from build123d import *

# Parameters (mm, degrees)
SKETCH1_W                = 120
SKETCH1_H                = 30
BOSS_EXTRUDE1_DEPTH      = 100
CUT_EXTRUDE1_DEPTH       = 121.415945788
CUT_EXTRUDE1_DEPTH_BACK  = 121.415945788
SKETCH2_R                = 2.15
SKETCH2_W                = 20.1
SKETCH2_H                = 40.4
SKETCH3_OUTSIDE_W        = 153.812
SKETCH3_OUTSIDE_H        = 133.812
CUT_EXTRUDE2_DEPTH       = 121.415945788
CUT_EXTRUDE3_START       = -30
CUT_EXTRUDE3_DEPTH       = 30
SKETCH5_W                = 67.698745078
SKETCH5_H                = 100.8
CUT_EXTRUDE4_DEPTH       = 26
RIB1_REACH               = 122.416
SKETCH6_WALL_W           = 284.590065176
SKETCH6_WALL_H           = 4
RIB6_REACH               = 122.416
SKETCH7_WALL_W           = 284.590065176
SKETCH7_WALL_H           = 4
BOSS_EXTRUDE2_DEPTH      = 5
BOSS_EXTRUDE2_DEPTH_BACK = 4
SKETCH8_R                = 2.15
CUT_EXTRUDE5_DEPTH       = 84.326168543
CUT_EXTRUDE5_DEPTH_BACK  = 84.326168543
SKETCH9_R                = 2.75
SKETCH10_R               = 5
CUT_EXTRUDE6_DEPTH       = 3
CHAMFER1_SIZE            = 8
CUT_EXTRUDE7_START       = -12.194246874
CUT_EXTRUDE7_DEPTH       = 12.194246874
SKETCH12_W               = 37.282730079
SKETCH12_H               = 58.292887361
CUT_EXTRUDE8_DEPTH       = 108.591821251
SKETCH13_W               = 20.1
SKETCH13_H               = 40.4
BOSS_EXTRUDE3_DEPTH      = 4
SKETCH16_W               = 60
SKETCH16_H               = 40
BOSS_EXTRUDE4_DEPTH      = 4
CUT_EXTRUDE9_DEPTH       = 109.484577329
CUT_EXTRUDE9_DEPTH_BACK  = 109.484577329
SKETCH14_R               = 2.75
SKETCH15_R               = 5
CUT_EXTRUDE10_DEPTH      = 2
CHAMFER2_SIZE            = 0.2
CHAMFER3_SIZE            = 10
CUT_EXTRUDE11_DEPTH      = 109.484577329
CUT_EXTRUDE11_DEPTH_BACK = 109.484577329
CHAMFER4_SIZE            = 10


# Read off the part's stored shape, not the designer's step: Cut-Extrude3, Cut-Extrude7
with BuildPart() as part:
    # Sketch1 → Boss-Extrude1 (new body)
    with BuildSketch(Plane(origin=(0, 0, 0), x_dir=(1, 0, 0), z_dir=(0, 1, 0))):
        with Locations((0, -15)):
            Rectangle(SKETCH1_W, SKETCH1_H)
    extrude(amount=BOSS_EXTRUDE1_DEPTH)

    # Sketch2 → Cut-Extrude1 (cut, two sides: drawn at the far end of the back side and taken through both)
    with BuildSketch(Plane.XY.offset(30).offset(-CUT_EXTRUDE1_DEPTH_BACK)):
        with Locations((-4.95, 82.583541889)):
            Circle(SKETCH2_R)
        with Locations((4.95, 82.583541889)):
            Circle(SKETCH2_R)
        with Locations((-4.95, 34.383541889)):
            Circle(SKETCH2_R)
        with Locations((4.95, 34.383541889)):
            Circle(SKETCH2_R)
        with Locations((0, 58.483541889)):
            Rectangle(SKETCH2_W, SKETCH2_H)
    extrude(amount=CUT_EXTRUDE1_DEPTH + CUT_EXTRUDE1_DEPTH_BACK, mode=Mode.SUBTRACT)

    # Sketch3 outside → Cut-Extrude2 (cut, through all)
    with BuildSketch(Plane.XY.offset(30)):
        with Locations((0, 50)):
            Rectangle(SKETCH3_OUTSIDE_W, SKETCH3_OUTSIDE_H)
        with BuildLine():
            Line((-45, 23.283541889), (45, 23.283541889))
            Line((45, 23.283541889), (19.804596008, 86.568297014))
            ThreePointArc((19.804596008, 86.568297014), (0, 100), (-19.804596008, 86.568297014))
            Line((-19.804596008, 86.568297014), (-45, 23.283541889))
        make_face(mode=Mode.SUBTRACT)
    extrude(amount=-CUT_EXTRUDE2_DEPTH, mode=Mode.SUBTRACT)

    # Cut-Extrude3 outline → Cut-Extrude3 (cut)
    with BuildSketch(Plane.XY.offset(30).offset(CUT_EXTRUDE3_START)):
        Polygon((30, 60.95991045), (30, 23.283541889), (45, 23.283541889), align=None)
        Polygon((-30, 23.283541889), (-30, 60.95991045), (-45, 23.283541889), align=None)
    extrude(amount=CUT_EXTRUDE3_DEPTH, mode=Mode.SUBTRACT)

    # Sketch5 → Cut-Extrude4 (cut)
    with BuildSketch(Plane.XY.offset(30)):
        with Locations((0, 78.683541889)):
            Rectangle(SKETCH5_W, SKETCH5_H)
    extrude(amount=-CUT_EXTRUDE4_DEPTH, mode=Mode.SUBTRACT)

    # Sketch6 wall → Rib1 (add, up to next)
    with BuildSketch(Plane(origin=(-30, 44.62172617, 17), x_dir=(0, -0.782514313837, 0.622632595228), z_dir=(0, 0.622632595228, 0.782514313837)), mode=Mode.PRIVATE) as rib1_sk1:
        with Locations((0, 2)):
            Rectangle(SKETCH6_WALL_W, SKETCH6_WALL_H)
    rib1_tool1 = extrude(rib1_sk1.sketch, amount=-RIB1_REACH, mode=Mode.PRIVATE) - part.part
    add(rib1_tool1.solids().sort_by_distance((-30, 44.62172617, 17))[0])

    # Sketch7 wall → Rib6 (add, up to next)
    with BuildSketch(Plane(origin=(30, 44.62172617, 17), x_dir=(0, -0.782514313837, 0.622632595228), z_dir=(0, -0.622632595228, -0.782514313837)), mode=Mode.PRIVATE) as rib6_sk1:
        with Locations((0, 2)):
            Rectangle(SKETCH7_WALL_W, SKETCH7_WALL_H)
    rib6_tool1 = extrude(rib6_sk1.sketch, amount=RIB6_REACH, mode=Mode.PRIVATE) - part.part
    add(rib6_tool1.solids().sort_by_distance((30, 44.62172617, 17))[0])

    # Sketch8 → Boss-Extrude2 (add, two sides: drawn at the far end of the back side and taken through both)
    with BuildSketch(Plane.XY.offset(4).offset(-BOSS_EXTRUDE2_DEPTH_BACK)):
        with Locations((-4.95, 82.583541889)):
            Circle(SKETCH8_R)
        with Locations((4.95, 82.583541889)):
            Circle(SKETCH8_R)
        with Locations((-4.95, 34.383541889)):
            Circle(SKETCH8_R)
        with Locations((4.95, 34.383541889)):
            Circle(SKETCH8_R)
    extrude(amount=BOSS_EXTRUDE2_DEPTH + BOSS_EXTRUDE2_DEPTH_BACK)

    # Sketch9 → Cut-Extrude5 (cut, two sides: drawn at the far end of the back side and taken through both)
    with BuildSketch(Plane(origin=(0, 28.283541889, 0), x_dir=(1, 0, 0), z_dir=(0, 1, 0)).offset(-CUT_EXTRUDE5_DEPTH_BACK)):
        with Locations(Location((-15, -15, 0), (0, 0, 270))):
            Circle(SKETCH9_R)
        with Locations(Location((15, -15, 0), (0, 0, 270))):
            Circle(SKETCH9_R)
    extrude(amount=CUT_EXTRUDE5_DEPTH + CUT_EXTRUDE5_DEPTH_BACK, mode=Mode.SUBTRACT)

    # Sketch10 → Cut-Extrude6 (cut)
    with BuildSketch(Plane(origin=(0, 28.283541889, 0), x_dir=(1, 0, 0), z_dir=(0, 1, 0))):
        with Locations(Location((-15, -15, 0), (0, 0, 270))):
            Circle(SKETCH10_R)
        with Locations(Location((15, -15, 0), (0, 0, 270))):
            Circle(SKETCH10_R)
    extrude(amount=-CUT_EXTRUDE6_DEPTH, mode=Mode.SUBTRACT)

    # Chamfer1
    # the kernel refuses this chamfer: 8 mm, written as the material it takes off along each edge
    with BuildSketch(Plane(origin=(-30, 2.710077985, 30), x_dir=(-0.02749587661058658, 0, -0.9996219169112968), z_dir=(0, 1, 0))) as chamfer1_piece_1:
        Polygon((CHAMFER1_SIZE * 0.999621916911, -CHAMFER1_SIZE * 0.0274958766106), (-CHAMFER1_SIZE * 0.0274958766106, -CHAMFER1_SIZE * 0.999621916911), (0, 0), align=None)
    extrude(amount=46.146927807, mode=Mode.SUBTRACT)
    with BuildSketch(Plane(origin=(30, 48.857005793, 30), x_dir=(-0.9996219169112968, 0, 0.027495876610586487), z_dir=(0, -1, 0))) as chamfer1_piece_2:
        Polygon((CHAMFER1_SIZE * 0.999621916911, CHAMFER1_SIZE * 0.0274958766106), (-CHAMFER1_SIZE * 0.0274958766106, CHAMFER1_SIZE * 0.999621916911), (0, 0), align=None)
    extrude(amount=46.146927807, mode=Mode.SUBTRACT)

    # Cut-Extrude7 outline → Cut-Extrude7 (cut)
    with BuildSketch(Plane.XZ.offset(-23.283541889).offset(CUT_EXTRUDE7_START)):
        with BuildLine():
            ThreePointArc((-27.724333118, 24.275666882), (-14.154563191, 28.553981218), (0, 30))
            Line((0, 30), (-22, 30))
            Line((-22, 30), (-27.724333118, 24.275666882))
        make_face()
        with BuildLine():
            ThreePointArc((0, 30), (14.154563191, 28.553981218), (27.724333118, 24.275666882))
            Line((27.724333118, 24.275666882), (22, 30))
            Line((22, 30), (0, 30))
        make_face()
    extrude(amount=CUT_EXTRUDE7_DEPTH, mode=Mode.SUBTRACT)

    # Sketch12 → Cut-Extrude8 (cut, through all)
    with BuildSketch(Plane.XY.offset(4)):
        with Locations((-0.669441285, 59.375969669)):
            Rectangle(SKETCH12_W, SKETCH12_H)
    extrude(amount=CUT_EXTRUDE8_DEPTH, mode=Mode.SUBTRACT)

    # Sketch13 → Boss-Extrude3 (add)
    with BuildSketch(Plane.XY.offset(4)):
        with Locations((0, 58.483541889)):
            Rectangle(SKETCH13_W, SKETCH13_H)
    extrude(amount=-BOSS_EXTRUDE3_DEPTH)

    # Sketch16 → Boss-Extrude4 (add)
    with BuildSketch(Plane(origin=(0, 0, 0), x_dir=(-1, 0, 0), z_dir=(0, 0, -1))):
        with Locations((0, 80.95991045)):
            Rectangle(SKETCH16_W, SKETCH16_H)
    extrude(amount=-BOSS_EXTRUDE4_DEPTH)

    # Sketch14 → Cut-Extrude9 (cut, two sides: drawn at the far end of the back side and taken through both)
    with BuildSketch(Plane.XY.offset(4).offset(-CUT_EXTRUDE9_DEPTH_BACK)):
        with Locations((0, 58.473541889)):
            Circle(SKETCH14_R)
    extrude(amount=CUT_EXTRUDE9_DEPTH + CUT_EXTRUDE9_DEPTH_BACK, mode=Mode.SUBTRACT)

    # Sketch15 → Cut-Extrude10 (cut)
    with BuildSketch(Plane.XY.offset(4)):
        with Locations((0, 58.473541889)):
            Circle(SKETCH15_R)
    extrude(amount=-CUT_EXTRUDE10_DEPTH, mode=Mode.SUBTRACT)

    # Chamfer2
    chamfer2_edges = [part.edges().sort_by_distance(p)[0] for p in [
        (-5, 58.473541889, 4),
    ]]
    chamfer(chamfer2_edges, length=CHAMFER2_SIZE)

    # Chamfer3
    chamfer3_edges = [part.edges().sort_by_distance(p)[0] for p in [
        (30, 100.95991045, 2),
        (-30, 100.95991045, 2),
    ]]
    chamfer(chamfer3_edges, length=CHAMFER3_SIZE)

    # Sketch17 → Cut-Extrude11 (cut, two sides: drawn at the far end of the back side and taken through both)
    with BuildSketch(Plane.XY.offset(4).offset(-CUT_EXTRUDE11_DEPTH_BACK)):
        Polygon((-49.480687217, 83.283541889), (47.707933407, 83.283541889), (47.707933407, 123.775741613), (-59.194126739, 121.253008662), align=None)
    extrude(amount=CUT_EXTRUDE11_DEPTH + CUT_EXTRUDE11_DEPTH_BACK, mode=Mode.SUBTRACT)

    # Chamfer4
    chamfer4_edges = [part.edges().sort_by_distance(p)[0] for p in [
        (-30, 83.283541889, 2),
        (30, 83.283541889, 2),
    ]]
    chamfer(chamfer4_edges, length=CHAMFER4_SIZE)


solid = part.part
Design review of the part built by this model. Coordinates are the model's own, in mm. A direction names the side the tool comes from. Round coordinates to 2 decimals unless told otherwise and drop trailing zeros. Loops run counter-clockwise (first coordinate to the right, second up) from the corner with the lowest first, then second, coordinate; pieces in that order, holes last. Notation, with made-up numbers: (-37, 4.5) -> (10, 4.5) arc R15 ccw to (10, 27.5) -> close; hole circle Ø4 at (64.5, 41.5). An arc over 180 degrees is marked (long way). Use one line per item in the form item = value. Start each with the question number.
Q1. Machinability: for faces 1 (the face through (12.8, 25.284, 17.2)), 2 (the face through (-30, 42, 8)), 3 (the face through (0, 28.284, 17)), which of the approach directions +Z, -Z, +X, -X, +Y, -Y give a long, thin tool a straight path to every point of the face, cutting with its end or side? Answer none if there is none.
Q2. We need section C-C on z = 15. Give the boundary of the cut face in (x, y).
Q3. Draft analysis for pull direction Y (two halves, no side actions). For faces 4 (the face through (-29, 31, 23)), 5 (the face through (2, 56, 2)), 6 (the face through (24.93, 78.354, 2.028)), 7 (the face through (-1.08, 53.59, 2.91)), state which applies: +Y half, -Y half, draft (parallel to the pull), parting line (faces both ways), or undercut.
Q4. We need section A-A on x = 15. Give the boundary of the cut face in (y, z).
Q5. We need section D-D on z = 5. Give the boundary of the cut face in (x, y), then the cut area to 3 significant figures.
Q6. We need section B-B on y = 39.5. Give the boundary of the cut face in (x, z), then the cut area to 3 significant figures.
Q7. Wall thickness on line 1 along X through (y, z) = (25, 15); line 2 along X through (y, z) = (26, 15); line 3 along X through (y, z) = (35.5, 11): over which ranges is each line inside the solid? List them lowest first. Write a range as [from, to].
Q8. For pin 1 Ø8 at (x, y) = (0, 58.47) entering from +Z; pin 2 Ø5 at (x, z) = (14, 16.5) entering from +Y; pin 3 Ø2 at (x, y) = (0, 42.5) entering from +Z; pin 4 Ø6.5 at (y, z) = (48.5, 19) entering from -X, all flat-tipped, find the tip position at first contact; note any pin that passes through.
Calculated:
q1.face_1 = +Y
q1.face_2 = +Z, -Z, -X, +Y, -Y
q1.face_3 = +Z, +Y
q2.outline = (-30, 23.28) -> (-17.75, 23.28) -> (-17.75, 25.28) -> (-20, 25.28) -> (-20, 28.28) -> (-26, 28.28) -> (-26, 47.14) -> (-30, 47.14) -> close; (-12.25, 23.28) -> (12.25, 23.28) -> (12.25, 25.28) -> (10, 25.28) -> (10, 28.28) -> (-10, 28.28) -> (-10, 25.28) -> (-12.25, 25.28) -> close; (17.75, 23.28) -> (30, 23.28) -> (30, 47.14) -> (26, 47.14) -> (26, 28.28) -> (20, 28.28) -> (20, 25.28) -> (17.75, 25.28) -> close
q3.face_4 = draft
q3.face_5 = undercut
q3.face_6 = +Y half
q3.face_7 = undercut
q4.outline = (23.28, 0) -> (83.28, 0) -> (83.28, 4) -> (28.28, 4) -> (28.28, 10) -> (25.28, 10) -> (25.28, 12.25) -> (23.28, 12.25) -> close; (23.28, 17.75) -> (25.28, 17.75) -> (25.28, 20) -> (28.28, 20) -> (28.28, 28.37) -> (23.28, 28.37) -> close
q5.outline = (-30, 23.28) -> (30, 23.28) -> (30, 59.7) -> (26, 59.7) -> (26, 28.28) -> (-26, 28.28) -> (-26, 59.7) -> (-30, 59.7) -> close
q5.area = 551 mm²
q6.outline = (-30, 0) -> (30, 0) -> (30, 21.08) -> (26, 21.08) -> (26, 4) -> (-26, 4) -> (-26, 21.08) -> (-30, 21.08) -> close
q6.area = 377 mm²
q7.line_1 = [-30, -17.75], [-12.25, 12.25], [17.75, 30]
q7.line_2 = [-30, -20], [-10, 10], [20, 30]
q7.line_3 = [-30, -26], [26, 30]
q8.pin_1 = 2
q8.pin_2 = 25.28
q8.pin_3 = 4
q8.pin_4 = through
